```python
from build123d import *

# Parameters (mm, degrees)
SKETCH2_W           = 4.5
SKETCH2_H           = 4.5
SKETCH2_W_2         = 10
SKETCH2_H_2         = 15
BOSS_EXTRUDE1_DEPTH = 2.25


with BuildPart() as part:
    # Sketch2 → Boss-Extrude1 (new body, symmetric)
    with BuildSketch(Plane.XY):
        with Locations((0, 17.25)):
            Rectangle(SKETCH2_W, SKETCH2_H)
        with Locations((0, 7.5)):
            Rectangle(SKETCH2_W_2, SKETCH2_H_2)
    extrude(amount=BOSS_EXTRUDE1_DEPTH, both=True)

    # Mirror1: part across plane


with BuildPart() as part_1:
    add(part.part)
    add(part.part.mirror(Plane.ZX))


solid = part_1.part
```
Input: part model. Units: mm. Frame: model coordinates. A direction names the side the tool comes from. Give positions to 0.01 mm unless a question says otherwise; leave off trailing zeros. Order: outer loops, then holes, each group sorted by start corner. A loop starts at its lowest first (then second) coordinate and runs counter-clockwise, first axis right, second up.
1. Set-up query: faces 1 (the face through (-2.25, -17, 0)), 2 (the face through (-4, 15, 0)), 3 (the face through (4, -15, 0)), 4 (the face through (2.25, 17, 0)). Return all of +Z, -Z, +X, -X, +Y, -Y with unobstructed straight access to the full face (end or side cutting, diameter ignored); none if empty.
Computed:
face 1: +Z, -Z, -X, -Y
face 2: +Z, -Z, -X, +Y
face 3: +Z, -Z, +X, -Y
face 4: +Z, -Z, +X, +Y
2. Pin query (flat end, axial travel): pin 1 Ø2 at (x, z) = (4, 1) entering from +Y; pin 2 Ø0.8 at (x, z) = (4, 1) entering from -Y. Return the tip coordinate at first contact, or that it passes through.
Computed:
pin 1: stops at y = 15
pin 2: stops at y = -15
3. Cut plane A-A (z = 1.45). Return loops of the section in (x, y), and give its area (4 significant figures).
Computed:
outline: (-5, -15) - (-2.25, -15) - (-2.25, -19.5) - (2.25, -19.5) - (2.25, -15) - (5, -15) - (5, 15) - (2.25, 15) - (2.25, 19.5) - (-2.25, 19.5) - (-2.25, 15) - (-5, 15) - close
area: 340.5 mm2
4. Cut plane C-C (x = 3.75). Return loops of the section in (y, z).
Computed:
outline: (-15, -2.25) - (15, -2.25) - (15, 2.25) - (-15, 2.25) - close
5. Line query: probe 1 along Y at (x, z) = (-4, -0.5). Output: solid intervals per line, ascending.
Computed:
probe 1: y = -15 to 15
6. Cut plane B-B (y = 16). Return loops of the section in (x, z).
Computed:
outline: (-2.25, -2.25) - (2.25, -2.25) - (2.25, 2.25) - (-2.25, 2.25) - close
